For this review, use the dimensioned drawing (mm, ordinates from the lowest corner) and the shaded views. Coordinates: 2 decimals unless noted, no trailing zeros. Loops run counter-clockwise (first coordinate to the right, second up) from the corner with the lowest first, then second, coordinate; pieces in that order, holes last.
1. Clearance check with a flat-ended pin moving along its axis: P1, Ø6, axis at x = 43.5, y = 15, coming from the -Z side. State where the tip first meets the part, or that it passes through.
2. Take a section at A-A, the plane y = 15. State the section outline as (x, z) points, then the cut area to 3 significant figures.
3. Take a section at B-B, the plane x = 43.5. State the section outline as (y, z) points.
4. To check wall thickness, follow probe 1 along Y at (x, z) = (43, 0.5); probe 2 along X at (y, z) = (15.75, 3.5); probe 3 along X at (y, z) = (11.5, 3.5). State the ranges of each line that lie inside material, in increasing order.
5. Take a section at C-C, the plane z = 2. State the section outline as (x, y) points.
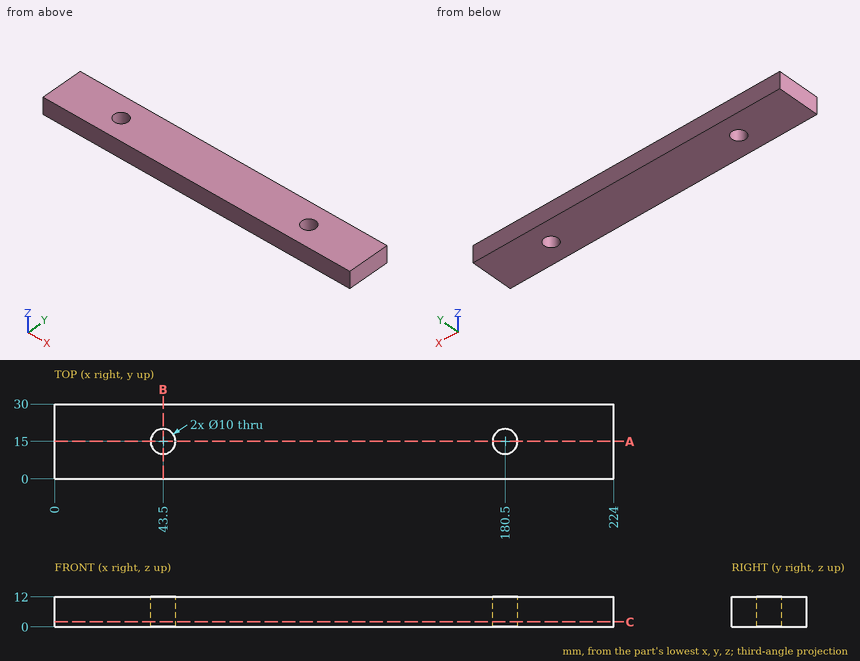
Results list:
1. P1: passes through
2. outline: (0, 0) - (38.5, 0) - (38.5, 12) - (0, 12) - close; (48.5, 0) - (175.5, 0) - (175.5, 12) - (48.5, 12) - close; (185.5, 0) - (224, 0) - (224, 12) - (185.5, 12) - close
2. area: 2,450 mm2
3. outline: (0, 0) - (10, 0) - (10, 12) - (0, 12) - close; (20, 0) - (30, 0) - (30, 12) - (20, 12) - close
4. probe 1: y = 0 to 10.03, 19.97 to 30
4. probe 2: x = 0 to 38.56, 48.44 to 175.56, 185.44 to 224
4. probe 3: x = 0 to 39.93, 47.07 to 176.93, 184.07 to 224
5. outline: (0, 0) - (224, 0) - (224, 30) - (0, 30) - close; hole circle Ø10 at (43.5, 15); hole circle Ø10 at (180.5, 15)
